Read the model definition and answer for the solid it produces. Units are mm, in the model's axes. A direction names the side the tool comes from. Coordinates: 2 decimals unless noted, no trailing zeros. Loops run counter-clockwise (first coordinate to the right, second up) from the corner with the lowest first, then second, coordinate; pieces in that order, holes last. Notation, with made-up numbers: (29.5, 72.5) - (84.5, 72.5) arc R34 ccw to (84.5, 108.5) - close; hole circle Ø11 at (6.5, 44.5). An arc over 180 degrees is marked (long way). Use one line per item in the form item = value.
from build123d import *

# Parameters (mm, degrees)
SKETCH_R        = 17
PAD_DEPTH       = 7
SKETCH002_R     = 15
SKETCH002_R_2   = 5
POCKET_DEPTH    = 5
SKETCH001_R     = 3
POCKET001_DEPTH = 5
SKETCH003_R     = 1
POCKET002_DEPTH = 5
CHAMFER_SIZE    = 1


with BuildPart() as part:
    # Sketch → Pad (new body)
    with BuildSketch(Plane.XY):
        Circle(SKETCH_R)
    extrude(amount=PAD_DEPTH)

    # Sketch002 → Pocket (cut)
    with BuildSketch(Plane.XY):
        Circle(SKETCH002_R)
        Circle(SKETCH002_R_2, mode=Mode.SUBTRACT)
    extrude(amount=POCKET_DEPTH, mode=Mode.SUBTRACT)

    # Sketch001 → Pocket001 (cut)
    with BuildSketch(Plane.XY):
        Circle(SKETCH001_R)
    extrude(amount=POCKET001_DEPTH, mode=Mode.SUBTRACT)

    # Sketch003 (on Face3 of Pocket001) → Pocket002 (cut)
    with BuildSketch(Plane.XY.offset(7)):
        with Locations((-9.109988, 7.483499)):
            Circle(SKETCH003_R)
    extrude(amount=-POCKET002_DEPTH, mode=Mode.SUBTRACT)

    # Chamfer
    chamfer_edges = [part.edges().sort_by_distance(p)[0] for p in [
        (-17, 0, 7),
    ]]
    chamfer(chamfer_edges, length=CHAMFER_SIZE)


solid = part.part
Item 1: For a pull along Y with two mould halves and no side action, classify faces 1 (the cylindrical face through (-1.08, -4.88, 2.46)), 2 (the flat face through (0, 0, 7)), 3 (the cylindrical face through (9.139, 14.334, 2.958)) as +Y half, -Y half, draft (parallel to the pull), parting line (faces both ways), or undercut.
Results below:
face_1 = undercut
face_2 = draft
face_3 = parting line
Item 2: The part is cut by section A-A on z = 2.5. Give the vertices of the cut face in (x, y), plus the area to 3 significant figures.
Results below:
outline = circle Ø34 at (0, 0); circle Ø10 at (0, 0); hole circle Ø30 at (0, 0); hole circle Ø6 at (0, 0)
area = 251 mm²
Item 3: Which of the six approach directions +Z, -Z, +X, -X, +Y, -Y give full straight-line access (tool end or side, diameter ignored) to faces 4 (the cylindrical face through (-8.186, 7.1, 6.014)), 5 (the flat face through (-4, 4, 5))?
Results below:
face_4 = +Z, -Z
face_5 = -Z
Item 4: The part is cut by section B-B on y = 0. Give the vertices of the cut face in (x, z), plus the area to 3 significant figures.
Results below:
outline = (-17, 0) - (-15, 0) - (-15, 5) - (-5, 5) - (-5, 0) - (-3, 0) - (-3, 5) - (3, 5) - (3, 0) - (5, 0) - (5, 5) - (15, 5) - (15, 0) - (17, 0) - (17, 6) - (16, 7) - (-16, 7) - (-17, 6) - close
area = 107 mm²
Item 5: Find the intervals of material crossed by L1, parallel to Y at x = 0, z = 2.35; L2, parallel to Y at x = -4.5, z = 2; L3, parallel to Y at x = 1, z = 2.5, in increasing order.
Results below:
L1 = -17 to -15, -5 to -3, 3 to 5, 15 to 17
L2 = -16.39 to -14.31, -2.18 to 2.18, 14.31 to 16.39
L3 = -16.97 to -14.97, -4.9 to -2.83, 2.83 to 4.9, 14.97 to 16.97
Item 6: Each of these flat-tipped pins is pushed along its axis until it touches: P1, Ø2, axis at x = 6, z = 2, coming from the +Y side; P2, Ø5, axis at x = 0, y = 0, coming from the -Z side; P3, Ø3, axis at y = 13.5, z = 4.5, coming from the +X side. Where does it stop, or does it pass through?
Results below:
P1 = 16.25
P2 = 5
P3 = 12.04
